CAD build for the part. Positions are in the model's coordinates, mm. Face numbers are marked on the shaded views. A direction names the side the tool comes from. Round coordinates to 2 decimals unless told otherwise and drop trailing zeros. Write each loop counter-clockwise with the first axis right and the second up, starting at its lowest first coordinate (ties: lowest second). Pieces come first, ordered by that corner, then holes. Notation, with made-up numbers: (9.25, 59.5) -> (52.25, 59.5) arc R20 cw to (52.25, 71.5) -> close; hole circle Ø10 at (30.25, 71). An arc over 180 degrees is marked (long way). Put each result on its own line as item: value. Start each with the question number.
1. 3-axis set-ups, long thin cutter, end or side, ignore diameter. For the marked faces 1, 2 and 3: which of +Z, -Z, +X, -X, +Y, -Y reach the whole face in a straight line?
2. Pull direction Y, two halves, no side cores. Call the marked faces 4, 5 and 6: pulls with the +Y half, pulls with the -Y half, needs draft (parallel to the pull), parting line crosses it, or undercut.
3. Saw through at A-A on y = -61.5. List the corners of the cut face in (x, z), and give its area (3 significant figures).
4. Flat gauge pins, fed straight in: P1, Ø18, axis at x = -10, y = 14, coming from the +Z side; P2, Ø18, axis at x = 13, y = 10, coming from the -Z side; P3, Ø2, axis at x = 39.5, z = 7.5, coming from the +Y side; P4, Ø18, axis at x = 0, y = 0, coming from the +Z side. Where does each tip first touch, or does it go through?
5. Drill centre lines: line 1 (X direction, y = 0, z = 3); line 2 (Y direction, x = 0, z = 5.5); line 3 (X direction, y = 0, z = 7). Where is each one in solid material? Low to high. Write a range as from..to.
6. Saw through at B-B on x = -61. State how many separate pieces and enclosed holes the cut face has, and give its area (3 significant figures).
7. Saw through at C-C on y = -39. List the corners of the cut face in (x, z).
from build123d import *

# Parameters (mm, degrees)
F1_DEPTH      = 10
F3_ANGLE      = 30
F5_COUNT      = 6
F6_R          = 30
F6_R_2        = 15
F7_DEPTH      = 12.8
F7_DEPTH_BACK = 4
F8_R          = 15
F9_DEPTH      = 25
F9_DEPTH_BACK = 25


with BuildPart() as f1:
    # F0 (on Top) → F1 (new body)
    with BuildSketch(Plane.XY):
        with BuildLine():
            Line((96.5925826289, 25.8819045103), (0, 0))
            Line((0, 0), (96.5925826289, -25.8819045103))
            ThreePointArc((96.5925826289, -25.8819045103), (100, 0), (96.5925826289, 25.8819045103))
        make_face()
    extrude(amount=F1_DEPTH)


with BuildPart() as f1_1:
    # F3: moved
    add(f1.part.rotate(Axis((55.2566722035, 0, 0), (1, 0, 0)), F3_ANGLE))

    # F5: F1 ×6 about axis
    f5_axis = Axis((0, 0, 15.24533052), (0, 0, 1))


with BuildPart() as f1_2:
    add(f1_1.part)
    for i in range(1, F5_COUNT):
        add(f1_1.part.rotate(f5_axis, i * 360 / F5_COUNT))

    # F6 (on Top) → F7 (join, two sides)
    with BuildSketch(Plane.XY) as f7_sk:
        Circle(F6_R)
        Circle(F6_R_2, mode=Mode.SUBTRACT)
    extrude(amount=F7_DEPTH)
    extrude(f7_sk.sketch, amount=-F7_DEPTH_BACK)

    # F8 (on Top) → F9 (cut, two sides)
    with BuildSketch(Plane.XY) as f9_sk:
        Circle(F8_R)
    extrude(amount=-F9_DEPTH, mode=Mode.SUBTRACT)
    extrude(f9_sk.sketch, amount=F9_DEPTH_BACK, mode=Mode.SUBTRACT)


solid = f1_2.part
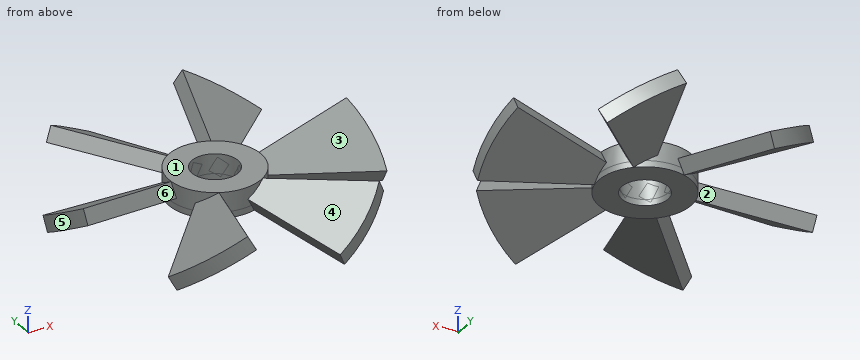
Return value:
1. face 1: +Z
1. face 2: -Z
1. face 3: +Z, +X
2. face 4: pulls with the -Y half
2. face 5: parting line crosses it
2. face 6: undercut
3. outline: (-64.15, -2.77) -> (-57.48, -10.99) -> (-18.73, 8.39) -> (-23.82, 17.39) -> close; (13.64, 0.61) -> (18.73, -8.39) -> (57.48, 10.99) -> (50.81, 19.2) -> close
3. area: 895 mm^2
4. P1: stops at z = 12.8
4. P2: stops at z = -4
4. P3: stops at y = 91.99
4. P4: passes through
5. line 1: x = -99.99..-15, 15..99.99
5. line 2: y = -30..-15, 15..30
5. line 3: x = -99.94..-15, 15..99.94
6. separate pieces: 3
6. enclosed holes: 0
6. area: 639 mm^2
7. outline: (-43.12, 1.25) -> (-36.45, -6.97) -> (-11.88, 5.32) -> (-16.97, 14.32) -> close; (6.78, 3.68) -> (11.88, -5.32) -> (36.45, 6.97) -> (29.78, 15.18) -> close
